Build history of the part. All positions in model axes, mm. Give positions to 0.01 mm unless a question says otherwise; leave off trailing zeros. Order: outer loops, then holes, each group sorted by start corner. A loop starts at its lowest first (then second) coordinate and runs counter-clockwise, first axis right, second up. Notation, with made-up numbers: (78.5, 63) - (88.5, 63) arc R22 cw to (88.5, 71) - close; hole circle Ø5 at (19, 66.5). An arc over 180 degrees is marked (long way). Answer in a Markdown table with one row per item.
```python
from build123d import *

# Parameters (mm, degrees)
SALIENTE_EXTRUIR1_DEPTH = 4
CROQUIS2_R              = 6.5
CORTAR_EXTRUIR1_DEPTH   = 4


with BuildPart() as part:
    # Croquis1 → Saliente-Extruir1 (new body)
    with BuildSketch(Plane.XY):
        with BuildLine():
            Line((0, 0), (10, 0))
            Line((10, 0), (10, 4))
            Line((10, 4), (25, 4))
            Line((25, 4), (25, 0))
            Line((25, 0), (35, 0))
            Line((35, 0), (35, 4))
            Line((35, 4), (50, 4))
            Line((50, 4), (50, 0))
            Line((50, 0), (60, 0))
            Line((60, 0), (60, 4))
            Line((60, 4), (75, 4))
            Line((75, 4), (75, 0))
            Line((75, 0), (85, 0))
            Line((85, 0), (85, 40))
            ThreePointArc((85, 40), (42.5, 82.5), (0, 40))
            Line((0, 40), (0, 0))
        make_face()
    extrude(amount=SALIENTE_EXTRUIR1_DEPTH)

    # Croquis2 → Cortar-Extruir1 (cut)
    with BuildSketch(Plane.XY.offset(4)):
        with Locations((42.5, 58)):
            Circle(CROQUIS2_R)
    extrude(amount=-CORTAR_EXTRUIR1_DEPTH, mode=Mode.SUBTRACT)


solid = part.part
```
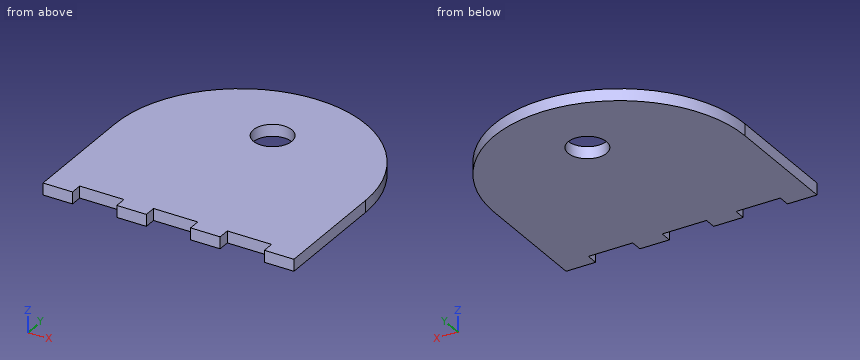
1. Cut at D-D on x = 12. Write the cut outline in (y, z).
Check result:
| item | result |
|---|---|
| outline | (4, 0) - (69.6, 0) - (69.6, 4) - (4, 4) - close |
2. Probe line 1 (Y direction, x = 42.5, z = 3.1); line 2 (Y direction, x = 38.5, z = 0.65); line 3 (X direction, y = 53, z = 0.65). List the from-to ranges inside material, lowest first.
Check result:
| item | result |
|---|---|
| line 1 | y = 4 to 51.5, 64.5 to 82.5 |
| line 2 | y = 4 to 52.88, 63.12 to 82.31 |
| line 3 | x = 2.04 to 38.35, 46.65 to 82.96 |
3. Drop a flat-ended pin along its axis: P1, Ø10.5, axis at x = 42.5, y = 58, coming from the -Z side. Give the stop position or say it passes through.
Check result:
| item | result |
|---|---|
| P1 | passes through |
4. Cut at C-C on z = 2.6. Write the cut outline in (x, y), and give its area (3 significant figures).
Check result:
| item | result |
|---|---|
| outline | (0, 0) - (10, 0) - (10, 4) - (25, 4) - (25, 0) - (35, 0) - (35, 4) - (50, 4) - (50, 0) - (60, 0) - (60, 4) - (75, 4) - (75, 0) - (85, 0) - (85, 40) arc R42.5 ccw to (0, 40) - close; hole circle Ø13 at (42.5, 58) |
| area | 5,920 mm² |
5. Cut at A-A on y = 58. Write the cut outline in (x, z), and give its area (3 significant figures).
Check result:
| item | result |
|---|---|
| outline | (4, 0) - (36, 0) - (36, 4) - (4, 4) - close; (49, 0) - (81, 0) - (81, 4) - (49, 4) - close |
| area | 256 mm² |
6. Cut at B-B on x = 42.5. Write the cut outline in (y, z), and give its area (3 significant figures).
Check result:
| item | result |
|---|---|
| outline | (4, 0) - (51.5, 0) - (51.5, 4) - (4, 4) - close; (64.5, 0) - (82.5, 0) - (82.5, 4) - (64.5, 4) - close |
| area | 262 mm² |
